Could you check a few things on this model? Use its own coordinates, in mm. Coordinates: 2 decimals unless noted, no trailing zeros. Use CSV: the item, a comma, the result in double quotes.
from build123d import *

# Parameters (mm, degrees)
F0_W     = 530
F0_H     = 80
F1_DEPTH = 30
F2_R     = 3
F3_DEPTH = 12
F4_R     = 3
F5_DEPTH = 12
F6_R     = 3
F7_DEPTH = 12
F8_R     = 3
F9_DEPTH = 12


with BuildPart() as f1:
    # F0 (on Right) → F1 (new body)
    with BuildSketch(Plane.YZ):
        with Locations((265, 40)):
            Rectangle(F0_W, F0_H)
    extrude(amount=F1_DEPTH)

    # F2 (on face) → F3 (cut)
    with BuildSketch(Plane(origin=(0, 0, 0), x_dir=(1, 0, 0), z_dir=(0, 0, -1))):
        with Locations((15, -130)):
            Circle(F2_R)
    extrude(amount=-F3_DEPTH, mode=Mode.SUBTRACT)

    # F4 (on face) → F5 (cut)
    with BuildSketch(Plane.XY.offset(80)):
        with Locations((15, 130)):
            Circle(F4_R)
    extrude(amount=-F5_DEPTH, mode=Mode.SUBTRACT)

    # F6 (on face) → F7 (cut)
    with BuildSketch(Plane(origin=(0, 0, 0), x_dir=(1, 0, 0), z_dir=(0, 0, -1))):
        with Locations((15, -400)):
            Circle(F6_R)
    extrude(amount=-F7_DEPTH, mode=Mode.SUBTRACT)

    # F8 (on face) → F9 (cut)
    with BuildSketch(Plane.XY.offset(80)):
        with Locations((15, 400)):
            Circle(F8_R)
    extrude(amount=-F9_DEPTH, mode=Mode.SUBTRACT)


solid = f1.part
(1) Please list where these lines run through material, in increasing order: line 1 (Y direction, x = 15, z = 8); line 2 (X direction, y = 130, z = 7).
Computed:
line 1,"y = 0 to 127, 133 to 397, 403 to 530"
line 2,"x = 0 to 12, 18 to 30"
(2) Will these pins go through, and if not, where does the flat tip stop? pin 1 (5.5 mm diameter, centred on x = 15, y = 130, fed in from -Z); pin 2 (3 mm diameter, centred on x = 14, y = 400, fed in from +Z).
Computed:
pin 1,"stops at z = 12"
pin 2,"stops at z = 68"
(3) Thinking about a two-plate mould opening in Y: for faces 1 (the face through (0, 261, 41)), 2 (the face through (15, 530, 39)), 3 (the face through (15, 0, 39)), which applies, +Y half, -Y half, draft (parallel to the pull), parting line (faces both ways), or undercut?
Computed:
face 1,"draft"
face 2,"+Y half"
face 3,"-Y half"
